from build123d import *

# Parameters (mm, degrees)
IZIM1_R                     = 7
IZIM1_R_2                   = 2.212355073
Y_KSEKLIK_EKSTR_ZYON1_DEPTH = 2
IZIM2_R                     = 3.5
IZIM2_R_2                   = 2.212355073
Y_KSEKLIK_EKSTR_ZYON2_DEPTH = 5
IZIM3_R                     = 1
KES_EKSTR_ZYON1_DEPTH       = 5
SCALE1_SCALE                = 0.666666667


with BuildPart() as part:
    # Çizim1 → Yükseklik-Ekstrüzyon1 (new body)
    with BuildSketch(Plane.XY):
        with Locations((-30.711927379, -38.904760786)):
            Circle(IZIM1_R)
        with Locations((-30.711927379, -38.904760786)):
            Circle(IZIM1_R_2, mode=Mode.SUBTRACT)
    extrude(amount=Y_KSEKLIK_EKSTR_ZYON1_DEPTH)

    # Çizim2 → Yükseklik-Ekstrüzyon2 (add)
    with BuildSketch(Plane.XY.offset(2)):
        with Locations((-30.711927379, -38.904760786)):
            Circle(IZIM2_R)
        with Locations((-30.711927379, -38.904760786)):
            Circle(IZIM2_R_2, mode=Mode.SUBTRACT)
    extrude(amount=-Y_KSEKLIK_EKSTR_ZYON2_DEPTH)

    # Çizim3 → Kes-Ekstrüzyon1 (cut)
    with BuildSketch(Plane(origin=(0, 0, 0), x_dir=(-1, 0, 0), z_dir=(0, 0, -1))):
        with Locations((30.711927379, -34.154760786)):
            Circle(IZIM3_R)
        with Locations((34.825548047, -41.279760786)):
            Circle(IZIM3_R)
        with Locations((26.598306711, -41.279760786)):
            Circle(IZIM3_R)
    extrude(amount=-KES_EKSTR_ZYON1_DEPTH, mode=Mode.SUBTRACT)


with BuildPart() as part_1:
    # Scale1: scaled about (-30.711927379, -38.904760786, 0.470967588)
    add(part.part.scale(SCALE1_SCALE).moved(Location((-10.237309126, -12.968253595, 0.156989196))))


solid = part_1.part
CAD build for the part. Positions are in the model's coordinates, mm. Coordinates: 2 decimals unless noted, no trailing zeros. Write each loop counter-clockwise with the first axis right and the second up, starting at its lowest first coordinate (ties: lowest second). Pieces come first, ordered by that corner, then holes. Notation, with made-up numbers: M 53,-12 L 109,-12 A18 ccw 109,16 Z; hole C 5,60.25 d8. An arc over 180 degrees is marked long. Answer as a JSON object with one key per item and string values. Group by question number.
1) Mould opens along Y. For faces 1 (the face through (-27.44, -40.89, 0.81)), 2 (the face through (-29, -41, 0.157)), 3 (the face through (-33, -40, 1)), 4 (the face through (-28.557, -39.798, -0.829)) say: +Y half, -Y half, draft (parallel to the pull), parting line (faces both ways), or undercut.
2) Saw through at A-A (x = -29.5). Write the cut outline in (y, z), plus the area to 3 significant figures.
3) Saw through at C-C (y = -40). Write the cut outline in (x, z), plus the area to 3 significant figures.
4) Saw through at B-B (y = -41). Write the cut outline in (x, z), plus the area to 3 significant figures.
5) Saw through at D-D (z = 1.3). Write the cut outline in (x, y), plus the area to 3 significant figures.
6) Pin check, flat tip, straight feed: pin 1 Ø1 at (y, z) = (-37, -1.5) entering from +X. Stop position of the tip, or through.
7) Wall check: line 1 (Z direction, x = -32.75, y = -41); line 2 (X direction, y = -38, z = -0.55); line 3 (Y direction, x = -29.5, z = -1.5). Give the ranges that are in metal, low to high. Write a range as from..to.
Values follow:
{
 "1": {"face 1": "undercut", "face 2": "draft", "face 3": "undercut", "face 4": "parting line"},
 "2": {"outline": "M -43.41,0.16 L -40.9,0.16 L -40.9,-1.84 L -39.75,-1.84 L -39.75,1.49 L -43.41,1.49 Z; M -38.06,-1.84 L -36.91,-1.84 L -36.91,0.16 L -34.4,0.16 L -34.4,1.49 L -38.06,1.49 Z", "area": "14.4 mm2"},
 "3": {"outline": "M -35.25,0.16 L -33.91,0.16 L -33.91,1.49 L -35.25,1.49 Z; M -33,0.16 L -32.77,0.16 L -32.77,-1.84 L -31.7,-1.84 L -31.7,1.49 L -33,1.49 Z; M -29.72,-1.84 L -28.65,-1.84 L -28.65,0.16 L -28.42,0.16 L -28.42,1.49 L -29.72,1.49 Z; M -27.52,0.16 L -26.18,0.16 L -26.18,1.49 L -27.52,1.49 Z", "area": "11.3 mm2"},
 "4": {"outline": "M -34.88,0.16 L -33.88,0.16 L -33.88,1.49 L -34.88,1.49 Z; M -33.03,0.16 L -31.74,0.16 L -31.74,-1.84 L -29.69,-1.84 L -29.69,0.16 L -28.4,0.16 L -28.4,1.49 L -33.03,1.49 Z; M -27.54,0.16 L -26.54,0.16 L -26.54,1.49 L -27.54,1.49 Z", "area": "12.9 mm2"},
 "5": {"outline": "C -30.71,-38.9 d9.33; hole C -33.45,-40.49 d1.33; hole C -30.71,-38.9 d2.95; hole C -30.71,-35.74 d1.33; hole C -27.97,-40.49 d1.33", "area": "57.4 mm2"},
 "6": {"pin 1": "stops at x = -28.85"},
 "7": {"line 1": "z = 0.16..1.49", "line 2": "x = -32.86..-31.88, -29.55..-28.56", "line 3": "y = -40.9..-39.75, -38.06..-36.91"}
}
